Autodesk Inventor part; units mm, degrees
ref_plane "Work Plane1" through (29, 0, 0) normal (0, -1, 0) x (1, 0, 0)
ref_plane "YZ Plane" through (0, 0, 0) normal (1, 0, 0) x (0, 1, 0)
ref_plane "XZ Plane" through (0, 0, 0) normal (0, 1, 0) x (-1, 0, 0)
sketch "Sketch1" plane through (0, 0, 0) normal (0, 0, 1) x (1, 0, 0)
  line L0 (0.2879, 0) -> (25.4, 0)
  line L1 (25.4, 0) -> (25.4, 2.413)
  line L2 (25.4, 2.413) -> (2.0322, 2.413)
  line L3 (2.0322, 2.413) -> (0.0001, 2.413)
  line L4 (0.0001, 2.413) -> (0, 2.413)
  line L5 (0, 2.413) -> (0, 4.5847)
  line L6 (0, 4.5847) -> (-2.5654, 4.5847)
  line L7 (-2.5654, 4.5847) -> (-2.5654, 1.8624)
  line L8 (-2.5654, 1.8624) -> (-0.7874, 1.8624)
  line L9 (-0.7874, 1.8624) -> (0.2879, 0)
  line L10 (-8.1585, 0) -> (30.9931, 0)
  line L11 (0, -0.9169) -> (0, 5.5016)
  line L12 (2.0322, 2.413) -> (0, 2.413) construction
  dimension "d1" = 23.3678
  dimension "d2" = 2.0321
  dimension "d3" = 2.5654
  dimension "d4" = 1.778
  dimension "d5" = 60
  dimension "d6" = 4.826
  dimension "d7" = 4.826
  dimension "d8" = 3.7248
  dimension "d9" = 9.1694
  dimension "d26" = 25.4
revolve "Body" add sketch "Sketch1" angle 360 about axis through (0.2879, 0, 0) along (1, 0, 0) contours L9 L11 L3 L2 L1 L0 | L9 L8 L7 L6 L5 L11
sketch "Sketch2" plane through (-2.5654, 0, 0) normal (-1, 0, 0) x (0, 0, 1)
  circle A0 centre (0, 0) radius 1.8624
  line L0 (0, -6.4186) -> (0, 6.4186)
  line L1 (-6.4186, 0) -> (6.4186, 0)
  line L2 (1.8624, 0) -> (0.9312, -1.6129)
  line L3 (0.9312, -1.6129) -> (-0.9312, -1.6129)
  line L4 (-0.9312, -1.6129) -> (-1.8624, 0)
  line L5 (-1.8624, 0) -> (-0.9312, 1.6129)
  line L6 (-0.9312, 1.6129) -> (0.9312, 1.6129)
  line L7 (0.9312, 1.6129) -> (1.8624, 0)
extrude "Slot" add sketch "Sketch2" against normal up to next contours L7 A0 | A0 L2 | L6 L0 A0 | A0 L0 L3 | L0 L6 A0 | A0 L3 L0 | L4 A0 | A0 L5
fillet "Fillet1" radius 1.778 1 edges at (-2.5654, -4.5847, 0)
thread "Thread"
chamfer "Chamfer1" distance 0.6492 distance2 0.6492 1 edges at (25.4, -2.413, 0) measured on face at (25.4, 0.9527, 0.2826)
ref_plane "Work Plane1" through (29, 0, 0) normal (0, -1, 0) x (1, 0, 0)
fillet "Fillet2" radius 0.1 1 edges at (0.0001, -2.413, 0)
equation "\"d30\" = R"
equation "\"d17\" = RR"
equation "\"d13\" = GEL"
equation "\"d15\" = -0.5 * SPD + 0.5 * GD"
equation "\"d16\" = GUL"
equation "\"d1\" = GEL"
equation "\"d3\" = KOH"
equation "\"d4\" = INTI"
equation "\"d6\" = GD"
equation "\"d7\" = BDM"
equation "\"d8\" = 1.1547 * SW"
equation "\"d9\" = KOD"
equation "\"d26\" = NLG"
equation "\"GD\" = NND"
equation "\"NLG\" = 25.4"
equation "\"GEL\" = 23.3678"
equation "\"KOD\" = 9.1694"
equation "\"KOH\" = 2.5654"
equation "\"INTI\" = 1.778"
equation "\"GAL\" = 2.032"
equation "\"GUL\" = 0.64922"
equation "\"BDM\" = NND"
equation "\"SW\" = 3.2258"
equation "\"RR\" = 1.778"
equation "\"SPD\" = GD1"
equation "\"R\" = 0.1"
equation "\"KR\" = 5.4102"
equation "\"GD1\" = 3.52755"
equation "\"THREADDIA\" = 4.826"
equation "\"FAWI\" = 45deg"
equation "\"KOH1\" = 1.778"
equation "\"NND\" = 4.826"
equation "\"TOA\" = 30deg"
equation "\"E0\" = 1.155 * SW"
properties part number "Unbrako - 10 x 1" material "Steel, Mild"
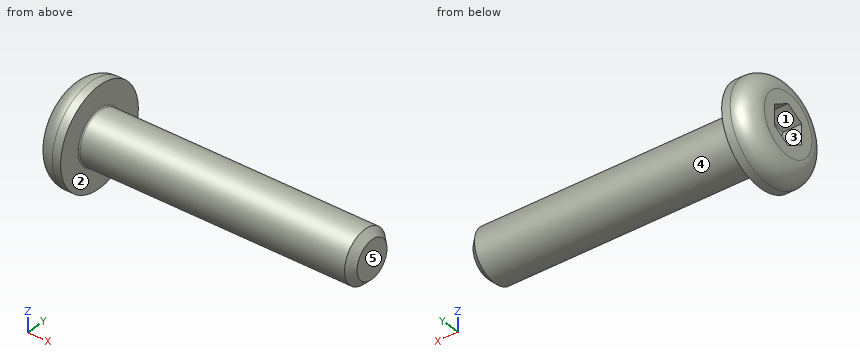
CAD build for the part. Positions are in the model's coordinates, mm. Face numbers are marked on the shaded views. A direction names the side the tool comes from. Coordinates: 2 decimals unless noted, no trailing zeros. Loops run counter-clockwise (first coordinate to the right, second up) from the corner with the lowest first, then second, coordinate; pieces in that order, holes last. Notation, with made-up numbers: (-30.75, 10.25) - (-24.75, 10.25) arc R17 ccw to (-24.75, 20.25) - close; hole circle Ø11 at (63, 23.25). An arc over 180 degrees is marked (long way). Use CSV: the item, a comma, the result in double quotes. Start each with the question number.
Q1. Cut at A-A, the plane x = 11.5. List the corners of the cut face in (y, z), then the cut area to 3 significant figures.
Q2. Drop flat-ended pins along their axis: P1, Ø5, axis at x = 0.5, z = -3, coming from the +Y side; P2, Ø0.9, axis at x = -1.5, z = -0.5, coming from the -Y side; P3, Ø2, axis at y = -2, z = -3, coming from the +X side. Give the stop position or say it passes through.
Q3. Probe probe 1 along Y at (x, z) = (7.25, 0); probe 2 along X at (y, z) = (-2.5, 2.5); probe 3 along X at (y, z) = (-2.5, -1). List the from-to ranges inside material, lowest first. Write a range as from..to.
Q4. Two-plate mould, pull along Z, no slides. Class the marked faces 3, 4 and 5: +Z half, -Z half, draft (parallel to the pull), parting line (faces both ways), or undercut.
Q5. 3-axis set-ups, long thin cutter, end or side, ignore diameter. For the marked faces 1 and 2: which of +Z, -Z, +X, -X, +Y, -Y reach the whole face in a straight line?
Here are the results:
1,outline,"circle Ø4.83 at (0, 0)"
1,area,"18.3 mm2"
2,P1,"y = 4.55"
2,P2,"y = -4.55"
2,P3,"x = 0"
3,probe 1,"-2.41..2.41"
3,probe 2,"-2.41..0"
3,probe 3,"-2.57..0"
4,face 3,"undercut"
4,face 4,"parting line"
4,face 5,"draft"
5,face 1,"-X"
5,face 2,"+X"
